```python
from build123d import *

# Parameters (mm, degrees)
SKETCH1_R           = 1.75
BOSS_EXTRUDE3_DEPTH = 4


with BuildPart() as part:
    # Sketch1 → Boss-Extrude3 (new body)
    with BuildSketch(Plane.XY):
        with BuildLine():
            ThreePointArc((11.398526221, 4), (3.187763399, 11.651805204), (-7.774744082, 9.245526186))
            ThreePointArc((-7.774744082, 9.245526186), (-8.865739978, 10.052419077), (-10.123446462, 10.561852666))
            ThreePointArc((-10.123446462, 10.561852666), (-10.344972209, 10.344972209), (-10.561852666, 10.123446462))
            ThreePointArc((-10.561852666, 10.123446462), (-10.052419077, 8.865739978), (-9.245526186, 7.774744082))
            ThreePointArc((-9.245526186, 7.774744082), (-9.583708351, 7.353838062), (-9.90274436, 6.918240682))
            ThreePointArc((-9.90274436, 6.918240682), (-11.16540472, 7.415268848), (-12.51210701, 7.581825517))
            ThreePointArc((-12.51210701, 7.581825517), (-12.669951657, 7.315), (-12.82210701, 7.044889767))
            ThreePointArc((-12.82210701, 7.044889767), (-12.004513558, 5.961889707), (-10.94274436, 5.116907842))
            ThreePointArc((-10.94274436, 5.116907842), (-11.160464753, 4.622815863), (-11.355888976, 4.119488508))
            ThreePointArc((-11.355888976, 4.119488508), (-12.704165582, 4.272780301), (-14.048088143, 4.085109489))
            ThreePointArc((-14.048088143, 4.085109489), (-14.131494839, 3.78652263), (-14.208555951, 3.486235477))
            ThreePointArc((-14.208555951, 3.486235477), (-13.138520279, 2.651746506), (-11.89423259, 2.110362789))
            ThreePointArc((-11.89423259, 2.110362789), (-11.976653925, 1.576756402), (-12.035148524, 1.04))
            ThreePointArc((-12.035148524, 1.04), (-13.377158555, 0.839108838), (-14.626715284, 0.31))
            ThreePointArc((-14.626715284, 0.31), (-14.63, 0), (-14.626715284, -0.31))
            ThreePointArc((-14.626715284, -0.31), (-13.377158555, -0.839108838), (-12.035148524, -1.04))
            ThreePointArc((-12.035148524, -1.04), (-11.976653925, -1.576756402), (-11.89423259, -2.110362789))
            ThreePointArc((-11.89423259, -2.110362789), (-13.138520279, -2.651746506), (-14.208555951, -3.486235477))
            ThreePointArc((-14.208555951, -3.486235477), (-14.131494839, -3.78652263), (-14.048088143, -4.085109489))
            ThreePointArc((-14.048088143, -4.085109489), (-12.704165582, -4.272780301), (-11.355888976, -4.119488508))
            ThreePointArc((-11.355888976, -4.119488508), (-11.160464753, -4.622815863), (-10.94274436, -5.116907842))
            ThreePointArc((-10.94274436, -5.116907842), (-12.004513558, -5.961889707), (-12.82210701, -7.044889767))
            ThreePointArc((-12.82210701, -7.044889767), (-12.669951657, -7.315), (-12.51210701, -7.581825517))
            ThreePointArc((-12.51210701, -7.581825517), (-11.16540472, -7.415268848), (-9.90274436, -6.918240682))
            ThreePointArc((-9.90274436, -6.918240682), (-9.583708351, -7.353838062), (-9.245526186, -7.774744082))
            ThreePointArc((-9.245526186, -7.774744082), (-10.052419077, -8.865739978), (-10.561852666, -10.123446462))
            ThreePointArc((-10.561852666, -10.123446462), (-10.344972209, -10.344972209), (-10.123446462, -10.561852666))
            ThreePointArc((-10.123446462, -10.561852666), (-8.865739978, -10.052419077), (-7.774744082, -9.245526186))
            ThreePointArc((-7.774744082, -9.245526186), (-7.353838062, -9.583708351), (-6.918240682, -9.90274436))
            ThreePointArc((-6.918240682, -9.90274436), (-7.415268848, -11.16540472), (-7.581825517, -12.51210701))
            ThreePointArc((-7.581825517, -12.51210701), (-7.315, -12.669951657), (-7.044889767, -12.82210701))
            ThreePointArc((-7.044889767, -12.82210701), (-5.961889707, -12.004513558), (-5.116907842, -10.94274436))
            ThreePointArc((-5.116907842, -10.94274436), (-4.622815863, -11.160464753), (-4.119488508, -11.355888976))
            ThreePointArc((-4.119488508, -11.355888976), (-4.272780301, -12.704165582), (-4.085109489, -14.048088143))
            ThreePointArc((-4.085109489, -14.048088143), (-3.78652263, -14.131494839), (-3.486235477, -14.208555951))
            ThreePointArc((-3.486235477, -14.208555951), (-2.651746506, -13.138520279), (-2.110362789, -11.89423259))
            ThreePointArc((-2.110362789, -11.89423259), (-1.576756402, -11.976653925), (-1.04, -12.035148524))
            ThreePointArc((-1.04, -12.035148524), (-0.839108838, -13.377158555), (-0.31, -14.626715284))
            ThreePointArc((-0.31, -14.626715284), (0, -14.63), (0.31, -14.626715284))
            ThreePointArc((0.31, -14.626715284), (0.839108838, -13.377158555), (1.04, -12.035148524))
            ThreePointArc((1.04, -12.035148524), (1.576756402, -11.976653925), (2.110362789, -11.89423259))
            ThreePointArc((2.110362789, -11.89423259), (2.651746506, -13.138520279), (3.486235477, -14.208555951))
            ThreePointArc((3.486235477, -14.208555951), (3.78652263, -14.131494839), (4.085109489, -14.048088143))
            ThreePointArc((4.085109489, -14.048088143), (4.272780301, -12.704165582), (4.119488508, -11.355888976))
            ThreePointArc((4.119488508, -11.355888976), (4.622815863, -11.160464753), (5.116907842, -10.94274436))
            ThreePointArc((5.116907842, -10.94274436), (5.961889707, -12.004513558), (7.044889767, -12.82210701))
            ThreePointArc((7.044889767, -12.82210701), (7.315, -12.669951657), (7.581825517, -12.51210701))
            ThreePointArc((7.581825517, -12.51210701), (7.415268848, -11.16540472), (6.918240682, -9.90274436))
            ThreePointArc((6.918240682, -9.90274436), (7.353838062, -9.583708351), (7.774744082, -9.245526186))
            ThreePointArc((7.774744082, -9.245526186), (8.865739978, -10.052419077), (10.123446462, -10.561852666))
            ThreePointArc((10.123446462, -10.561852666), (10.344972209, -10.344972209), (10.561852666, -10.123446462))
            ThreePointArc((10.561852666, -10.123446462), (10.052419077, -8.865739978), (9.245526186, -7.774744082))
            ThreePointArc((9.245526186, -7.774744082), (9.583708351, -7.353838062), (9.90274436, -6.918240682))
            ThreePointArc((9.90274436, -6.918240682), (11.16540472, -7.415268848), (12.51210701, -7.581825517))
            ThreePointArc((12.51210701, -7.581825517), (12.669951657, -7.315), (12.82210701, -7.044889767))
            ThreePointArc((12.82210701, -7.044889767), (12.004513558, -5.961889707), (10.94274436, -5.116907842))
            ThreePointArc((10.94274436, -5.116907842), (11.184585981, -4.564146845), (11.398526221, -4))
            Line((11.398526221, -4), (30.75, -4))
            ThreePointArc((30.75, -4), (34.75, 0), (30.75, 4))
            Line((30.75, 4), (11.398526221, 4))
        make_face()
        Circle(SKETCH1_R, mode=Mode.SUBTRACT)
        with Locations((30.75, 0)):
            Circle(SKETCH1_R, mode=Mode.SUBTRACT)
    extrude(amount=BOSS_EXTRUDE3_DEPTH)


solid = part.part
```
Design review of the part built by this model. Coordinates are the model's own, in mm. A direction names the side the tool comes from. Give positions to 0.01 mm unless a question says otherwise; leave off trailing zeros. Order: outer loops, then holes, each group sorted by start corner. A loop starts at its lowest first (then second) coordinate and runs counter-clockwise, first axis right, second up. Notation, with made-up numbers: M 81,71 L 90,71 A20 cw 90,90 Z; hole C 83.5,-23.5 d11. An arc over 180 degrees is marked long. One line per question, with ' | ' between items. Start each with the question number.
Q1. We need section B-B (y = -8.75). Write out the cut boundary in (x, z).
Q2. The part is to be moulded in two halves that separate along X. For faces 6 (the face through (21, -4, 2)), 7 (the face through (-8.88, -10.06, 1.97)), 8 (the face through (-11.991, -5.948, 1.972)), say which applies: +X half, -X half, draft (parallel to the pull), parting line (faces both ways), or undercut.
Q3. We need section A-A (z = 2.15). State how many separate pieces and enclosed holes the cut face has, plus the area to 3 significant figures.
Q4. For L1, parallel to Y at x = 30.75, z = 2.45; L2, parallel to Y at x = 0, z = 1.9; L3, parallel to Y at x = 27, z = 3.4, list the stretches that pass through material, from the lowest coordinate up. Write a range as [from, to].
Q5. We need section C-C (y = 6). Write out the cut boundary in (x, z), plus the area to 3 significant figures.
Q6. For pin 1 Ø1 at (y, z) = (8.5, 3) entering from +X; pin 2 Ø1 at (y, z) = (8, 1) entering from -X; pin 3 Ø4.5 at (x, y) = (30.75, 0) entering from -Z; pin 4 Ø1.2 at (x, z) = (24, 1) entering from -Y, all flat-tipped, find the tip position at first contact; note any pin that passes through.
Q7. Machinability: for faces 1 (the face through (-8.849, 10.043, 1.972)), 2 (the face through (8.849, -10.043, 1.972)), 3 (the face through (-11.978, -1.569, 1.972)), 4 (the face through (4, -1, 4)), 5 (the face through (-11.1, 7.4, 2)), which of the approach directions +Z, -Z, +X, -X, +Y, -Y give a long, thin tool a straight path to every point of the face, cutting with its end or side? Answer none if there is none.
Returned:
1) outline: M -9.99,0 L 9.99,0 L 9.99,4 L -9.99,4 Z
2) face 6: draft | face 7: undercut | face 8: -X half
3) separate pieces: 1 | enclosed holes: 2 | area: 672 mm2
4) L1: [-4, -1.75], [1.75, 4] | L2: [-14.63, -1.75], [1.75, 12.08] | L3: [-4, 4]
5) outline: M -12.04,0 L 10.48,0 L 10.48,4 L -12.04,4 Z | area: 90.1 mm2
6) pin 1: x = 9.05 | pin 2: x = -12.56 | pin 3: z = 0 | pin 4: y = -4
7) face 1: +Z, -Z, +Y | face 2: +Z, -Z, -Y | face 3: +Z, -Z, -X | face 4: +Z, +X, -X, +Y, -Y | face 5: +Z, -Z
